Check sheet for the modelled part. Datum: model origin and axes. Units: mm. Face numbers are marked on the shaded views. A direction names the side the tool comes from. Round coordinates to 2 decimals unless told otherwise and drop trailing zeros. Loops run counter-clockwise (first coordinate to the right, second up) from the corner with the lowest first, then second, coordinate; pieces in that order, holes last. Notation, with made-up numbers: (-37, 73.5) -> (8, 73.5) arc R11 ccw to (8, 91.5) -> close; hole circle Ø3 at (27, -39.5). An arc over 180 degrees is marked (long way). Return JSON: item names as keys, results as strings.
Autodesk Inventor part; units mm, degrees
ref_plane "BODY_N_XY" through (122, 0, 0) normal (0, 0, -1) x (1, 0, 0)
ref_plane "BODY_N_YZ" through (122, 0, 0) normal (1, 0, 0) x (0, -1, 0)
ref_plane "BODY_N_ZX" through (122, 0, 0) normal (0, -1, 0) x (0, 0, -1)
sketch "Sketch_8" plane through (0, 0, 0) normal (0, 0, 1) x (1, 0, 0)
  line L0 (0, 0) -> (-8, 0)
  line L1 (-8, 0) -> (-8, 4.3865)
  line L2 (-8, 4.3865) -> (-7.3865, 5)
  line L3 (-7.3865, 5) -> (0, 5)
  line L4 (0, 5) -> (0, 0)
  line L5 (0, 0) -> (-8, 0)
revolve "Revolution1" add sketch "Sketch_8" angle 360 about axis through (0, 0, 0) along (1, 0, 0)
thread "Thread1"
sketch "Sketch_9" plane through (0, 0, 0) normal (1, 0, 0) x (0, 0, -1)
  line L0 (-9.15, 4.0345) -> (-9.15, -4.0345)
  arc A0 (-9.15, -4.0345) -> (-4.0345, -9.15) centre (0, 0) ccw
  line L1 (-4.0345, -9.15) -> (4.0345, -9.15)
  arc A1 (4.0345, -9.15) -> (9.15, -4.0345) centre (0, 0) ccw
  line L2 (9.15, -4.0345) -> (9.15, 4.0345)
  arc A2 (9.15, 4.0345) -> (4.0345, 9.15) centre (0, 0) ccw
  line L3 (4.0345, 9.15) -> (-4.0345, 9.15)
  arc A3 (-4.0345, 9.15) -> (-9.15, 4.0345) centre (0, 0) ccw
extrude "Extrusion1" add sketch "Sketch_9" along normal blind 12.5
sketch "Sketch_11" plane through (12.5, 0, 0) normal (1, 0, 0) x (0, 0, -1)
  circle A0 centre (0, 0) radius 8.7
extrude "Extrusion2" add sketch "Sketch_11" along normal blind 100
sketch "Sketch_10" plane through (112.5, 0, 0) normal (1, 0, 0) x (0, 0, -1)
  line L0 (-9.15, 4.0345) -> (-9.15, -4.0345)
  arc A0 (-9.15, -4.0345) -> (-4.0345, -9.15) centre (0, 0) ccw
  line L1 (-4.0345, -9.15) -> (4.0345, -9.15)
  arc A1 (4.0345, -9.15) -> (9.15, -4.0345) centre (0, 0) ccw
  line L2 (9.15, -4.0345) -> (9.15, 4.0345)
  arc A2 (9.15, 4.0345) -> (4.0345, 9.15) centre (0, 0) ccw
  line L3 (4.0345, 9.15) -> (-4.0345, 9.15)
  arc A3 (-4.0345, 9.15) -> (-9.15, 4.0345) centre (0, 0) ccw
extrude "Extrusion3" add sketch "Sketch_10" along normal blind 9.5
sketch "Sketch7" plane through (0, 0, 0) normal (0, 0, 1) x (1, 0, 0)
  line L0 (8, 9.15) -> (8, 4.15)
  line L1 (8, 2.9566) -> (5.933, 4.15)
  line L2 (5.933, 4.15) -> (5.933, 8.717)
  line L3 (5.933, 8.717) -> (5.5, 9.15)
  line L4 (5.5, 9.15) -> (8, 9.15)
  line L5 (8, 9.15) -> (8, 2.9566)
revolve "Revolution2" cut sketch "Sketch7" angle 360 about axis through (8, 9.15, 0) along (0, 1, 0)
thread "Thread2"
sketch "Sketch_7" plane through (0, 0, 0) normal (0, 0, 1) x (1, 0, 0)
  line L0 (117, 9.15) -> (117, 4.15)
  line L1 (117, 2.9566) -> (114.933, 4.15)
  line L2 (114.933, 4.15) -> (114.933, 8.717)
  line L3 (114.933, 8.717) -> (114.5, 9.15)
  line L4 (114.5, 9.15) -> (117, 9.15)
  line L5 (117, 9.15) -> (117, 2.9566)
revolve "Revolution3" cut sketch "Sketch_7" angle 360 about axis through (117, 9.15, 0) along (0, 1, 0)
thread "Thread3"
sketch "Sketch_16" plane through (0, 0, 0) normal (0, 0, 1) x (1, 0, 0)
  line L0 (92.5, 0) -> (-8, 0)
  line L1 (-8, 0) -> (-8, 2.5)
  line L2 (-8, 2.5) -> (12.5, 2.5)
  line L3 (12.5, 2.5) -> (12.5, 8)
  line L4 (12.5, 8) -> (92.5, 8)
  line L5 (92.5, 8) -> (92.5, 0)
  line L6 (92.5, 0) -> (-8, 0)
revolve "Revolution4" cut sketch "Sketch_16" angle 360 about axis through (92.5, 0, 0) along (1, 0, 0)
ref_plane "BODY_N_XY" through (122, 0, 0) normal (0, 0, -1) x (1, 0, 0)
ref_plane "BODY_N_YZ" through (122, 0, 0) normal (1, 0, 0) x (0, -1, 0)
ref_plane "BODY_N_ZX" through (122, 0, 0) normal (0, -1, 0) x (0, 0, -1)
ref_plane "NUT2_XY" through (122, 0, 0) normal (1, 0, 0) x (0, 0, -1)
ref_plane "NUT2_YZ" through (122, 0, 0) normal (0, 0, -1) x (0, 1, 0)
ref_plane "NUT2_ZX" through (122, 0, 0) normal (0, 1, 0) x (1, 0, 0)
ref_plane "SW1_XY" through (17.5, 0, 0) normal (1, 0, 0) x (0, 0, -1)
ref_plane "SW1_YZ" through (17.5, 0, 0) normal (0, 0, -1) x (0, 1, 0)
ref_plane "SW1_ZX" through (17.5, 0, 0) normal (0, 1, 0) x (1, 0, 0)
ref_plane "SW2_XY" through (107.5, 0, 0) normal (-1, 0, 0) x (0, 0, -1)
ref_plane "SW2_YZ" through (107.5, 0, 0) normal (0, 0, -1) x (0, -1, 0)
ref_plane "SW2_ZX" through (107.5, 0, 0) normal (0, -1, 0) x (-1, 0, 0)
ref_plane "SW_R1_XY" through (17.5, -14.15, 0) normal (1, 0, 0) x (0, 0, -1)
ref_plane "SW_R1_YZ" through (17.5, -14.15, 0) normal (0, 0, -1) x (0, 1, 0)
ref_plane "SW_R1_ZX" through (17.5, -14.15, 0) normal (0, 1, 0) x (1, 0, 0)
ref_plane "SW_R2_XY" through (107.5, -14.15, 0) normal (-1, 0, 0) x (0, 0, -1)
ref_plane "SW_R2_YZ" through (107.5, -14.15, 0) normal (0, 0, -1) x (0, -1, 0)
ref_plane "SW_R2_ZX" through (107.5, -14.15, 0) normal (0, -1, 0) x (-1, 0, 0)
ref_plane "body_XY" through (0, 0, 0) normal (1, 0, 0) x (0, 0, -1)
ref_plane "body_YZ" through (0, 0, 0) normal (0, 0, -1) x (0, 1, 0)
ref_plane "body_ZX" through (0, 0, 0) normal (0, 1, 0) x (1, 0, 0)
properties part number "CJ2B16-75Z(1_0)_BODY"
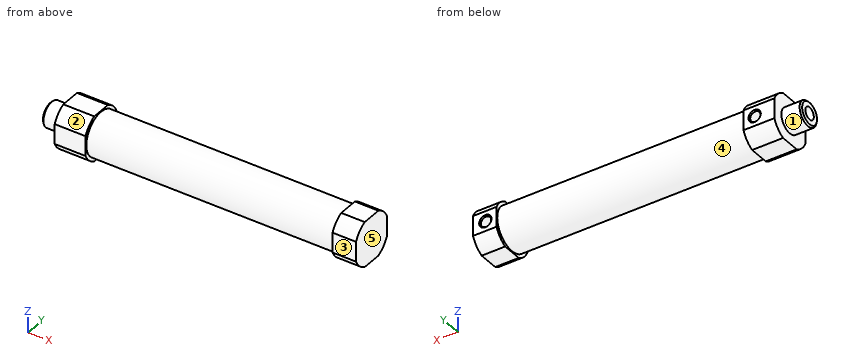
Q1. Section check D-D (x = 109.5). Record the boundary of the cut face in (y, z), then the cut area to 3 significant figures.
Results list:
{"outline": "circle Ø17.4 at (0, 0)", "area": "238 mm^2"}
Q2. Section check C-C (z = -6.25). Record the boundary of the cut face in (x, y).
Results list:
{"outline": "(0, -7.81) -> (12.5, -7.81) -> (12.5, -6.05) -> (112.5, -6.05) -> (112.5, -7.81) -> (122, -7.81) -> (122, 7.81) -> (112.5, 7.81) -> (112.5, 6.05) -> (12.5, 6.05) -> (12.5, 7.81) -> (0, 7.81) -> close; hole (12.5, -4.99) -> (92.5, -4.99) -> (92.5, 4.99) -> (12.5, 4.99) -> close"}
Q3. Section check A-A (y = 0). Record the boundary of the cut face in (x, z), then the cut area to 3 significant figures.
Results list:
{"outline": "(-8, -4.39) -> (-7.39, -5) -> (0, -5) -> (0, -9.15) -> (12.5, -9.15) -> (12.5, -8.7) -> (112.5, -8.7) -> (112.5, -9.15) -> (122, -9.15) -> (122, 9.15) -> (112.5, 9.15) -> (112.5, 8.7) -> (12.5, 8.7) -> (12.5, 9.15) -> (0, 9.15) -> (0, 5) -> (-7.39, 5) -> (-8, 4.39) -> (-8, 2.5) -> (12.5, 2.5) -> (12.5, 8) -> (92.5, 8) -> (92.5, -8) -> (12.5, -8) -> (12.5, -2.5) -> (-8, -2.5) -> close", "area": "840 mm^2"}
Q4. Material ranges on line 1 (X direction, y = -2.25, z = -1.75); line 2 (Z direction, x = -2.25, y = 0); line 3 (X direction, y = -1.5, z = 6.5), recorded low to high.
Results list:
{"line 1": "-8 to 12.5, 92.5 to 122", "line 2": "-5 to -2.5, 2.5 to 5", "line 3": "0 to 12.5, 92.5 to 122"}
Q5. Section check B-B (x = 23.5). Record the boundary of the cut face in (y, z).
Results list:
{"outline": "circle Ø17.4 at (0, 0); hole circle Ø16 at (0, 0)"}
Q6. Tool access check on the marked faces 1 and 2. Record the directions out of +Z, -Z, +X, -X, +Y, -Y that give a thin tool (end or side, any length) a straight path to the whole face; none if there is none.
Results list:
{"face 1": "-X", "face 2": "+Z, +X, -X, -Y"}
Q7. Go/stop test with flat-tipped pins: pin 1 (6 mm diameter, centred on x = 75, z = -0.5, fed in from -Y); pin 2 (6 mm diameter, centred on y = 0, z = 0, fed in from -X); pin 3 (3 mm diameter, centred on y = -6.5, z = 5.5, fed in from -X); pin 4 (3 mm diameter, centred on x = 7.5, y = 6, fed in from +Z). Record where each tip stops, or that it passes through.
Results list:
{"pin 1": "y = -8.7", "pin 2": "x = -8", "pin 3": "x = 0", "pin 4": "z = 8.93"}
Q8. Draft check along X on the marked faces 3, 4 and 5. Enter one of: released by +X, released by -X, zero draft, split by the parting line, or undercut.
Results list:
{"face 3": "zero draft", "face 4": "undercut", "face 5": "released by +X"}
